Verification items for the finished model (mm, model axes). Round coordinates to 2 decimals unless told otherwise and drop trailing zeros. Write each loop counter-clockwise with the first axis right and the second up, starting at its lowest first coordinate (ties: lowest second). Pieces come first, ordered by that corner, then holes. Notation, with made-up numbers: M 64.5,71 L 97.5,71 A9 cw 97.5,77 Z; hole C 14.5,9 d5. An arc over 180 degrees is marked long. One line per item, written item: value. Start each with the question number.
from build123d import *

# Parameters (mm, degrees)
SKETCH2_W                                        = 130
SKETCH2_H                                        = 130
BOSS_EXTRUDE1_DEPTH                              = 5
SKETCH3_R                                        = 13.5
CUT_EXTRUDE1_DEPTH                               = 5
SKETCH8_W                                        = 130
SKETCH8_H                                        = 130
CUT_EXTRUDE6_DEPTH                               = 6
M4_CLEARANCE_HOLE1_D                             = 4.8
M4_CLEARANCE_HOLE1_DEPTH                         = 5
CBORE_FOR_M3_HEX_HEAD_MACHINE_SCREW1_D           = 3.4
CBORE_FOR_M3_HEX_HEAD_MACHINE_SCREW1_DEPTH       = 5
CBORE_FOR_M3_HEX_HEAD_MACHINE_SCREW1_CBORE_D     = 6.5
CBORE_FOR_M3_HEX_HEAD_MACHINE_SCREW1_CBORE_DEPTH = 3.3
CBORE_FOR_M4_SBHCS1_D                            = 4.5
CBORE_FOR_M4_SBHCS1_DEPTH                        = 5
CBORE_FOR_M4_SBHCS1_CBORE_D                      = 8.6
CBORE_FOR_M4_SBHCS1_CBORE_DEPTH                  = 2.2


with BuildPart() as part:
    # Sketch2 → Boss-Extrude1 (new body)
    with BuildSketch(Plane(origin=(0, 0, 0), x_dir=(1, 0, 0), z_dir=(0, 1, 0))):
        Rectangle(SKETCH2_W, SKETCH2_H)
    extrude(amount=BOSS_EXTRUDE1_DEPTH)

    # Sketch3 → Cut-Extrude1 (cut)
    with BuildSketch(Plane(origin=(0, 5, 0), x_dir=(1, 0, 0), z_dir=(0, 1, 0))):
        Circle(SKETCH3_R)
    extrude(amount=-CUT_EXTRUDE1_DEPTH, mode=Mode.SUBTRACT)

    # Sketch8 → Cut-Extrude6 (cut, through all)
    with BuildSketch(Plane(origin=(0, 5, 0), x_dir=(1, 0, 0), z_dir=(0, 1, 0))):
        Rectangle(SKETCH8_W, SKETCH8_H)
        with BuildLine():
            Line((-42.00982343, 32.5), (42.00982343, 32.5))
            ThreePointArc((42.00982343, 32.5), (50.201409492, 28.235670649), (51.406671379, 19.079583559))
            Line((51.406671379, 19.079583559), (25.74494306, -51.420416441))
            ThreePointArc((25.74494306, -51.420416441), (22.083765761, -56.191586062), (16.348095112, -58))
            Line((16.348095112, -58), (-16.348095112, -58))
            ThreePointArc((-16.348095112, -58), (-22.083765761, -56.191586062), (-25.74494306, -51.420416441))
            Line((-25.74494306, -51.420416441), (-51.406671379, 19.079583559))
            ThreePointArc((-51.406671379, 19.079583559), (-50.201409492, 28.235670649), (-42.00982343, 32.5))
        make_face(mode=Mode.SUBTRACT)
    extrude(amount=-CUT_EXTRUDE6_DEPTH, mode=Mode.SUBTRACT)

    # M4 Clearance Hole1
    with Locations(Plane(origin=(0, 5, 0), x_dir=(1, 0, 0), z_dir=(0, 1, 0))):
        with Locations((-27, 24), (27, 24), (27, -24), (-27, -24)):
            Hole(M4_CLEARANCE_HOLE1_D / 2, depth=M4_CLEARANCE_HOLE1_DEPTH)

    # CBORE for M3 Hex Head Machine Screw1
    with Locations(Plane(origin=(0, 5, 0), x_dir=(1, 0, 0), z_dir=(0, 1, 0))):
        with Locations((-15.5, 15.5), (15.5, 15.5), (15.5, -15.5), (-15.5, -15.5)):
            CounterBoreHole(CBORE_FOR_M3_HEX_HEAD_MACHINE_SCREW1_D / 2, CBORE_FOR_M3_HEX_HEAD_MACHINE_SCREW1_CBORE_D / 2, CBORE_FOR_M3_HEX_HEAD_MACHINE_SCREW1_CBORE_DEPTH, depth=CBORE_FOR_M3_HEX_HEAD_MACHINE_SCREW1_DEPTH)

    # CBORE for M4 SBHCS1
    with Locations(Plane(origin=(0, 0, 0), x_dir=(-1, 0, 0), z_dir=(0, -1, 0))):
        with Locations((0, -46.19), (40, 23.1), (-40, 23.1)):
            CounterBoreHole(CBORE_FOR_M4_SBHCS1_D / 2, CBORE_FOR_M4_SBHCS1_CBORE_D / 2, CBORE_FOR_M4_SBHCS1_CBORE_DEPTH, depth=CBORE_FOR_M4_SBHCS1_DEPTH)


solid = part.part
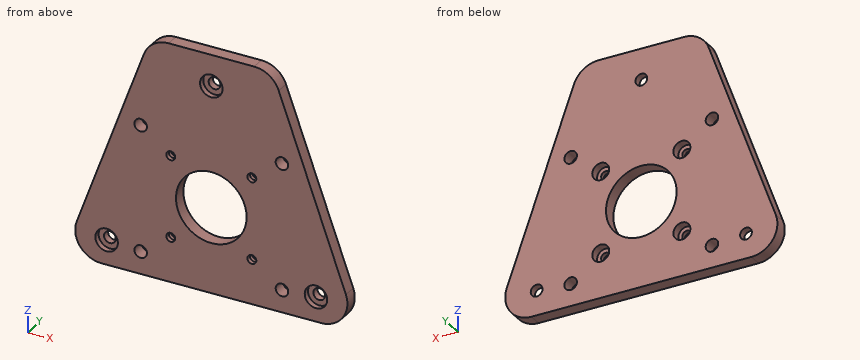
1) Cross-section at B-B (z = 0). Record the boundary of the cut face in (x, y), then the cut area to 3 significant figures.
2) Cross-section at A-A (z = -15.5). Record the boundary of the cut face in (x, y).
3) Cross-section at C-C (x = 11). Record the boundary of the cut face in (y, z).
4) Thickness scan on line 1 (Z direction, x = -15.5, y = 3.85); line 2 (Z direction, x = 0, y = 3.2); line 3 (X direction, y = 2.05, z = -24). Record the ranges inside material, lowest first.
5) Cross-section at D-D (z = 46.19). Record the boundary of the cut face in (x, y).
6) Gauge pin test, flat ends, axial feed: pin 1 Ø4 at (x, z) = (40, -23.1) entering from -Y; pin 2 Ø2.5 at (x, z) = (-38, -24.5) entering from -Y; pin 3 Ø1.5 at (y, z) = (2.5, 20.5) entering from +X; pin 4 Ø1 at (y, z) = (2, 32.5) entering from +X. Record the tip position at first contact, or that the pin passes through.
Results below:
1. outline: M -44.46,0 L -13.5,0 L -13.5,5 L -44.46,5 Z; M 13.5,0 L 44.46,0 L 44.46,5 L 13.5,5 Z
1. area: 310 mm²
2. outline: M -50.1,0 L -17.2,0 L -17.2,1.7 L -18.75,1.7 L -18.75,5 L -50.1,5 Z; M -13.8,0 L 13.8,0 L 13.8,1.7 L 12.25,1.7 L 12.25,5 L -12.25,5 L -12.25,1.7 L -13.8,1.7 Z; M 17.2,0 L 50.1,0 L 50.1,5 L 18.75,5 L 18.75,1.7 L 17.2,1.7 Z
3. outline: M 0,-32.5 L 5,-32.5 L 5,-7.83 L 0,-7.83 Z; M 0,7.83 L 5,7.83 L 5,58 L 0,58 Z
4. line 1: z = -32.5 to -18.75, -12.25 to 12.25, 18.75 to 58
4. line 2: z = -32.5 to -13.5, 13.5 to 43.94, 48.44 to 58
4. line 3: x = -51.9 to -44.2, -35.8 to -29.4, -24.6 to 24.6, 29.4 to 35.8, 44.2 to 51.9
5. outline: M -27.65,0 L -4.3,0 L -4.3,2.2 L -2.25,2.2 L -2.25,5 L -27.65,5 Z; M 2.25,2.2 L 4.3,2.2 L 4.3,0 L 27.65,0 L 27.65,5 L 2.25,5 Z
6. pin 1: passes through
6. pin 2: stops at y = 2.2
6. pin 3: stops at x = 37.27
6. pin 4: stops at x = 32.81
